Read the model definition and answer for the solid it produces. Units are mm, in the model's axes. A direction names the side the tool comes from. Coordinates: 2 decimals unless noted, no trailing zeros. Write each loop counter-clockwise with the first axis right and the second up, starting at its lowest first coordinate (ties: lowest second). Pieces come first, ordered by that corner, then holes.
1) The part is cut by section D-D (x = -86). Determine the outline of the cut face in (y, z), then the cut area to 3 significant figures.
2) Each of these flat-tipped pins is pushed along its axis until it touches: pin 1 Ø8.5 at (y, z) = (46, 23) entering from -X; pin 2 Ø5 at (y, z) = (38, 22) entering from +X; pin 3 Ø5 at (y, z) = (55, 10.5) entering from -X. Where does it stop, or does it pass through?
3) The part is cut by section B-B (z = 0). Determine the outline of the cut face in (x, y), then the cut area to 3 significant figures.
4) Find the intervals of material crossed by line 1 (X direction, y = 6.75, z = 0); line 2 (Y direction, x = 48, z = -24.75); line 3 (Z direction, x = 27, y = 54.5), in increasing order.
5) The part is cut by section C-C (y = 47). Give the number of separate pieces and of enclosed holes in the cut face, then the cut area to 3 significant figures.
6) The part is cut by section A-A (x = -48). Determine the outline of the cut face in (y, z), then the cut area to 3 significant figures.
7) Which of the six approach directions +Z, -Z, +X, -X, +Y, -Y give full straight-line access (tool end or side, diameter ignored) to faces 1 (the face through (-19, 54, -23)), 2 (the face through (-1, 33, -14.2)), 3 (the face through (-70, 43, -23)), 4 (the face through (70, 43, -23))?
8) Determine the mould class of faces 5 (the face through (-103.719, 22.594, -0.441)), 6 (the face through (41.506, 47.286, -22.971)), 7 (the face through (-1, 26, 31.5)) for opening direction X: +X half, -X half, draft (parallel to the pull), parting line (faces both ways), or undercut.
from build123d import *

# Parameters (mm, degrees)
SKETCH1_W           = 212
SKETCH1_H           = 63
SKETCH1_R           = 6.5
BOSS_EXTRUDE1_DEPTH = 25
SKETCH2_R           = 6.5
BOSS_EXTRUDE2_DEPTH = 17.3
FILLET1_R           = 8
FILLET2_R           = 5


with BuildPart() as part:
    # Sketch1 → Boss-Extrude1 (new body)
    with BuildSketch(Plane(origin=(0, 0, 0), x_dir=(1, 0, 0), z_dir=(0, 1, 0))):
        Rectangle(SKETCH1_W, SKETCH1_H)
        with Locations((86, 0)):
            Circle(SKETCH1_R, mode=Mode.SUBTRACT)
        with Locations((-86, 0)):
            Circle(SKETCH1_R, mode=Mode.SUBTRACT)
    extrude(amount=BOSS_EXTRUDE1_DEPTH)

    # Sketch2 → Boss-Extrude2 (add)
    with BuildSketch(Plane.XY.offset(31.5)):
        with BuildLine():
            Line((-70, 25), (70, 25))
            Line((70, 25), (70, 61))
            ThreePointArc((70, 61), (67.656854249, 66.656854249), (62, 69))
            Line((62, 69), (34, 69))
            Line((34, 69), (0, 35))
            Line((0, 35), (-34, 69))
            Line((-34, 69), (-62, 69))
            ThreePointArc((-62, 69), (-67.656854249, 66.656854249), (-70, 61))
            Line((-70, 61), (-70, 25))
        make_face()
        with Locations((-48, 47)):
            Circle(SKETCH2_R, mode=Mode.SUBTRACT)
        with Locations((48, 47)):
            Circle(SKETCH2_R, mode=Mode.SUBTRACT)
    boss_extrude2 = extrude(amount=-BOSS_EXTRUDE2_DEPTH)

    # Mirror1: Boss-Extrude2 across plane
    add(boss_extrude2.mirror(Plane.XY))

    # Fillet1
    fillet1_edges = [part.edges().sort_by_distance(p)[0] for p in [
        (-106, 25, 0),
        (106, 25, 0),
    ]]
    fillet(fillet1_edges, radius=FILLET1_R)

    # Fillet2
    fillet2_edges = [part.edges().sort_by_distance(p)[0] for p in [
        (0, 35, 22.85),
        (0, 35, -22.85),
    ]]
    fillet(fillet2_edges, radius=FILLET2_R)


solid = part.part
Reported:
1. outline: (0, -31.5) - (25, -31.5) - (25, -6.5) - (0, -6.5) - close; (0, 6.5) - (25, 6.5) - (25, 31.5) - (0, 31.5) - close
1. area: 1,250 mm2
2. pin 1: stops at x = -70
2. pin 2: stops at x = 70
2. pin 3: passes through
3. outline: (-106, 0) - (-92.5, 0) - (-92.5, 25) - (-98, 25) arc R8 ccw to (-106, 17) - close; (-79.5, 0) - (79.5, 0) - (79.5, 25) - (-79.5, 25) - close; (92.5, 0) - (106, 0) - (106, 17) arc R8 ccw to (98, 25) - (92.5, 25) - close
3. area: 4,620 mm2
4. line 1: x = -106 to -92.5, -79.5 to 79.5, 92.5 to 106
4. line 2: y = 0 to 40.5, 53.5 to 69
4. line 3: z = -31.5 to -14.2, 14.2 to 31.5
5. separate pieces: 8
5. enclosed holes: 0
5. area: 3,110 mm2
6. outline: (0, -31.5) - (40.5, -31.5) - (40.5, -14.2) - (25, -14.2) - (25, 14.2) - (40.5, 14.2) - (40.5, 31.5) - (0, 31.5) - close; (53.5, -31.5) - (69, -31.5) - (69, -14.2) - (53.5, -14.2) - close; (53.5, 14.2) - (69, 14.2) - (69, 31.5) - (53.5, 31.5) - close
6. area: 2,650 mm2
7. face 1: +Z, -Z, +Y
7. face 2: +X, -X, +Y
7. face 3: +Z, -Z, -X, +Y
7. face 4: +Z, -Z, +X, +Y
8. face 5: -X half
8. face 6: undercut
8. face 7: draft
